Study the drawing (mm; zero at the part's minimum x, y, z) and answer. A direction names the side the tool comes from. Coordinates: 2 decimals unless noted, no trailing zeros. Write each loop counter-clockwise with the first axis right and the second up, starting at its lowest first coordinate (ties: lowest second). Pieces come first, ordered by that corner, then holes. Notation, with made-up numbers: (-11, 78.25) -> (30, 78.25) arc R9 ccw to (30, 85.25) -> close; hole circle Ø2 at (77.25, 26.5). An arc over 180 degrees is marked (long way). Answer in a Markdown table with one row per item. Add a question column.
Item 1: Section C-C on y = 364 is taken. Write down the section's boundary in (x, z).
Item 2: Straight lines are drawn through the part: line 1 (Z direction, x = 49.5, y = 121); line 2 (Y direction, x = 395.5, z = 47.5). For each, find the intervals that lie inside material, in ascending order. Write a range as from..to.
Item 3: Which of the six approach directions +Z, -Z, +X, -X, +Y, -Y give full straight-line access (tool end or side, diameter ignored) to the marked faces 1 and 2?
Item 4: Section B-B on z = 104.5 is taken. Write down the section's boundary in (x, y).
Item 5: Section A-A on x = 139.5 is taken. Write down the section's boundary in (y, z), then the cut area to 3 significant figures.
Item 6: Given pin 1 Ø4 at (x, y) = (505, 456) entering from +Z, flat-ended and moving along its own axis, determine where the tip first touches the part or whether it passes through.
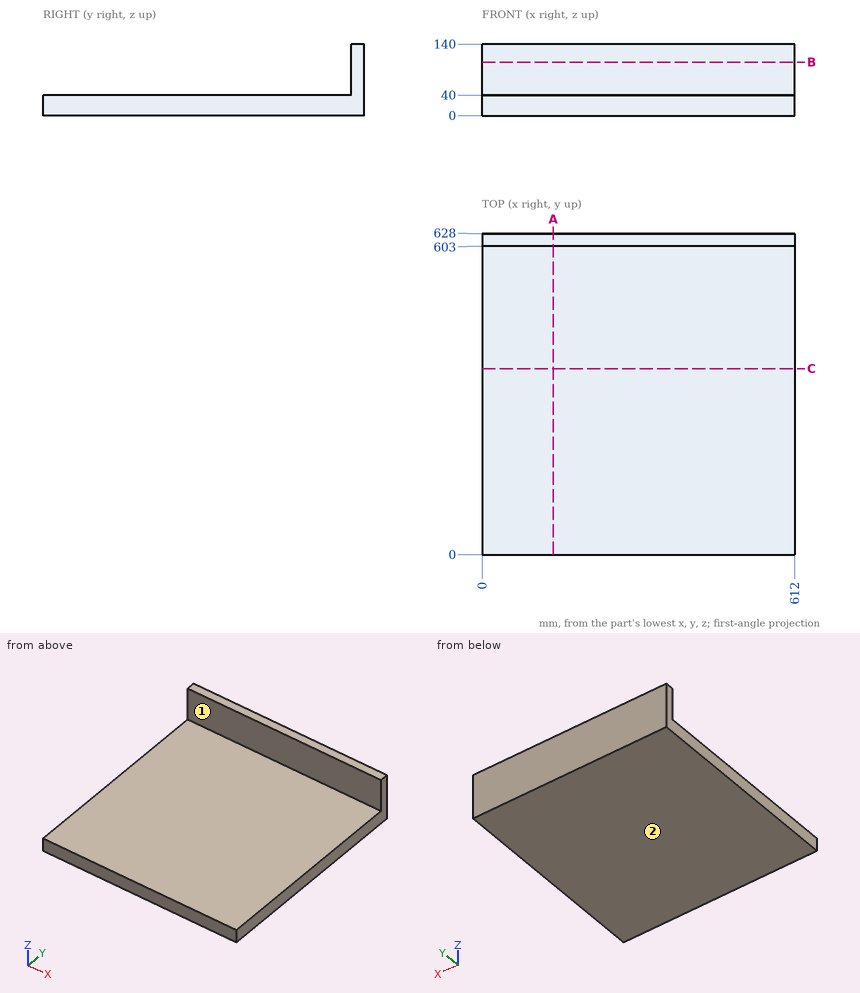
Results below:
| question | item | result |
|---|---|---|
| 1 | outline | (0, 0) -> (612, 0) -> (612, 40) -> (0, 40) -> close |
| 2 | line 1 | z = 0..40 |
| 2 | line 2 | y = 603..628 |
| 3 | face 1 | +Z, +X, -X, -Y |
| 3 | face 2 | -Z, +X, -X, +Y, -Y |
| 4 | outline | (0, 603) -> (612, 603) -> (612, 628) -> (0, 628) -> close |
| 5 | outline | (0, 0) -> (628, 0) -> (628, 140) -> (603, 140) -> (603, 40) -> (0, 40) -> close |
| 5 | area | 27,600 mm2 |
| 6 | pin 1 | stops at z = 40 |
